```python
from build123d import *

# Parameters (mm, degrees)
BOSS_EXTRUDE1_DEPTH = 10


with BuildPart() as part:
    # Sketch1 → Boss-Extrude1 (new body)
    with BuildSketch(Plane.XY):
        with BuildLine():
            Line((-25.4, -57.15), (-25.4, -28.26893))
            ThreePointArc((-25.4, -28.26893), (-27.259871939, -23.778801939), (-31.75, -21.91893))
            Line((-31.75, -21.91893), (-42.935289515, -21.91893))
            ThreePointArc((-42.935289515, -21.91893), (-49.274890295, -19.766942948), (-52.994414486, -14.200370743))
            ThreePointArc((-52.994414486, -14.200370743), (-54.864, 0), (-52.994414486, 14.200370743))
            ThreePointArc((-52.994414486, 14.200370743), (-49.274890295, 19.766942948), (-42.935289515, 21.91893))
            Line((-42.935289515, 21.91893), (-31.75, 21.91893))
            ThreePointArc((-31.75, 21.91893), (-27.259871939, 23.778801939), (-25.4, 28.26893))
            Line((-25.4, 28.26893), (-25.4, 57.15))
            ThreePointArc((-25.4, 57.15), (-24.47006403, 59.39506403), (-22.225, 60.325))
            Line((-22.225, 60.325), (22.225, 60.325))
            ThreePointArc((22.225, 60.325), (24.47006403, 59.39506403), (25.4, 57.15))
            Line((25.4, 57.15), (25.4, 28.26893))
            ThreePointArc((25.4, 28.26893), (27.259871939, 23.778801939), (31.75, 21.91893))
            Line((31.75, 21.91893), (42.935289515, 21.91893))
            ThreePointArc((42.935289515, 21.91893), (49.274890295, 19.766942948), (52.994414486, 14.200370743))
            ThreePointArc((52.994414486, 14.200370743), (54.864, 0), (52.994414486, -14.200370743))
            ThreePointArc((52.994414486, -14.200370743), (49.274890295, -19.766942948), (42.935289515, -21.91893))
            Line((42.935289515, -21.91893), (31.75, -21.91893))
            ThreePointArc((31.75, -21.91893), (27.259871939, -23.778801939), (25.4, -28.26893))
            Line((25.4, -28.26893), (25.4, -57.15))
            ThreePointArc((25.4, -57.15), (24.47006403, -59.39506403), (22.225, -60.325))
            Line((22.225, -60.325), (-22.225, -60.325))
            ThreePointArc((-22.225, -60.325), (-24.47006403, -59.39506403), (-25.4, -57.15))
        make_face()
    extrude(amount=BOSS_EXTRUDE1_DEPTH)


solid = part.part
```
Model file for the job. Use its own axes, mm. A direction names the side the tool comes from. Coordinates: 2 decimals unless noted, no trailing zeros. Write each loop counter-clockwise with the first axis right and the second up, starting at its lowest first coordinate (ties: lowest second). Pieces come first, ordered by that corner, then holes. Notation, with made-up numbers: (-37, -15.75) - (-27, -15.75) arc R15 ccw to (-27, -10.75) - close; hole circle Ø6 at (57.25, -23). An arc over 180 degrees is marked (long way). One line per question, with ' | ' between items. Start each with the question number.
Q1. Cut at B-B, the plane x = -40. List the corners of the cut face in (y, z).
Q2. Pin check, flat tips, straight feed: pin 1 (5 mm diameter, centred on x = 36.5, z = 6, fed in from +Y); pin 2 (6 mm diameter, centred on y = 48, z = 3, fed in from +X); pin 3 (6 mm diameter, centred on y = -7.5, z = 6, fed in from +X). Stop position of each tip, or through.
Q3. Cut at A-A, the plane z = 5.5. List the corners of the cut face in (x, y) (3 decimals), then the cut area to 3 significant figures.
Q4. Drill centre lines: line 1 (X direction, y = 41, z = 2.25); line 2 (Y direction, x = 44, z = 8); line 3 (Y direction, x = 28, z = 4). Where is each one in solid material? Low to high. Write a range as [from, to].
Q5. Cut at C-C, the plane y = -36. List the corners of the cut face in (x, z), then the cut area to 3 significant figures.
Q6. 3-axis set-ups, long thin cutter, end or side, ignore diameter. For faces 1 (the face through (-27.31, 23.73, 4.93)), 2 (the face through (37, 21.919, 5)), 3 (the face through (-37, -21.919, 5)), 4 (the face through (25.4, -43, 5)): which of +Z, -Z, +X, -X, +Y, -Y reach the whole face in a straight line?
Answer below:
1) outline: (-21.92, 0) - (21.92, 0) - (21.92, 10) - (-21.92, 10) - close
2) pin 1: y = 21.92 | pin 2: x = 25.4 | pin 3: x = 54.68
3) outline: (-52.994, -14.2) arc R10.414 ccw to (-42.935, -21.919) - (-31.75, -21.919) arc R6.35 cw to (-25.4, -28.269) - (-25.4, -57.15) arc R3.175 ccw to (-22.225, -60.325) - (22.225, -60.325) arc R3.175 ccw to (25.4, -57.15) - (25.4, -28.269) arc R6.35 cw to (31.75, -21.919) - (42.935, -21.919) arc R10.414 ccw to (52.994, -14.2) arc R54.864 ccw to (52.994, 14.2) arc R10.414 ccw to (42.935, 21.919) - (31.75, 21.919) arc R6.35 cw to (25.4, 28.269) - (25.4, 57.15) arc R3.175 ccw to (22.225, 60.325) - (-22.225, 60.325) arc R3.175 ccw to (-25.4, 57.15) - (-25.4, 28.269) arc R6.35 cw to (-31.75, 21.919) - (-42.935, 21.919) arc R10.414 ccw to (-52.994, 14.2) arc R54.864 ccw to start | area: 8,560 mm^2
4) line 1: [-25.4, 25.4] | line 2: [-21.86, 21.86] | line 3: [-23.14, 23.14]
5) outline: (-25.4, 0) - (25.4, 0) - (25.4, 10) - (-25.4, 10) - close | area: 508 mm^2
6) face 1: +Z, -Z, -X, +Y | face 2: +Z, -Z, +X, +Y | face 3: +Z, -Z, -X, -Y | face 4: +Z, -Z, +X, -Y
